For this review, take the finished solid that the model builds, in its own axes (mm). Face numbers are marked on the shaded views. A direction names the side the tool comes from. Give positions to 0.01 mm unless a question says otherwise; leave off trailing zeros. Loops run counter-clockwise (first coordinate to the right, second up) from the corner with the lowest first, then second, coordinate; pieces in that order, holes last. Notation, with made-up numbers: (-19, 74.5) - (30, 74.5) arc R31 cw to (30, 107.5) - close; hole circle Ø8 at (-10.75, -33.75). An arc over 180 degrees is marked (long way). Use CSV: the item, a comma, the result in double quotes. Start each with the question number.
1. For the marked faces 1, 2 and 3, list the 3-axis set-ups (+Z, -Z, +X, -X, +Y, -Y) from which the entire face can be reached by the end or side of a thin tool; tool diameter is ignored.
2. Take a section at B-B on x = -6.5. Give the boundary of the cut face in (y, z).
3. Take a section at A-A on z = 1.5. Give the boundary of the cut face in (x, y), plus the area to 3 significant figures.
4. Take a section at D-D on z = -1.5. Give the boundary of the cut face in (x, y), plus the area to 3 significant figures.
5. Wall thickness on line 1 (X direction, y = -4, z = -1.9); line 2 (Y direction, x = 7, z = 2.05); line 3 (X direction, y = -3.75, z = 0.25): over which ranges is each line inside the solid? List them lowest first.
6. Take a section at C-C on y = -3.5. Give the boundary of the cut face in (x, z).
7. For pin 1 (2.5 mm diameter, centred on x = -7, y = -4, fed in from -Z); pin 2 (3 mm diameter, centred on x = 9, y = -2.5, fed in from +Z); pin 3 (3 mm diameter, centred on x = 6, y = -4, fed in from +Z); pin 4 (2.5 mm diameter, centred on x = -7, y = -4, fed in from +Z), all flat-tipped, find the tip position at first contact; note any pin that passes through.
```python
from build123d import *

# Parameters (mm, degrees)
F1_DEPTH = 8
F3_D     = 2
F3_DEPTH = 0.6618861731
F4_D     = 2
F5_DEPTH = 1.5


with BuildPart() as f1:
    # F0 (on Front) → F1 (new body)
    with BuildSketch(Plane.XZ):
        with BuildLine():
            ThreePointArc((0.1467019637, 3.2967375591), (2.6022180015, 2.0293992886), (3.2331454446, -0.6608861731))
            Line((3.2331454446, -0.6608861731), (10.2443375631, -0.6608861731))
            Line((10.2443375631, -0.6608861731), (10.2443375631, 3.2967375591))
            Line((10.2443375631, 3.2967375591), (7.589418496, 3.2967375591))
            ThreePointArc((7.589418496, 3.2967375591), (5.7792360743, 3.6359179316), (4.2146449918, 4.6074417191))
            ThreePointArc((4.2146449918, 4.6074417191), (0, 6.2443375631), (-4.2146449918, 4.6074417191))
            ThreePointArc((-4.2146449918, 4.6074417191), (-5.7792360743, 3.6359179316), (-7.589418496, 3.2967375591))
            Line((-7.589418496, 3.2967375591), (-10.2443375631, 3.2967375591))
            Line((-10.2443375631, 3.2967375591), (-10.2443375631, -0.6608861731))
            Line((-10.2443375631, -0.6608861731), (-3.2331454446, -0.6608861731))
            ThreePointArc((-3.2331454446, -0.6608861731), (-2.6022180015, 2.0293992886), (-0.1467019637, 3.2967375591))
            ThreePointArc((-0.1467019637, 3.2967375591), (0, 3.3), (0.1467019637, 3.2967375591))
        make_face()
    extrude(amount=F1_DEPTH)

    # F3 (through all, one way)
    with BuildSketch(Plane.XY):
        with Locations((-7, -4), (7, -4)):
            Circle(F3_D / 2)
    extrude(amount=-F3_DEPTH, mode=Mode.SUBTRACT)

    # F4 (through all)
    with Locations(Plane(origin=(0, 0, 0), x_dir=(1, 0, 0), z_dir=(0, 0, -1))):
        with Locations((-7, 4), (7, 4)):
            Hole(F4_D / 2)

    # F5 (add): faces of the model
    f5_faces = [f1.faces().sort_by_distance(p)[0] for p in [
        (3.3395206367, -4, -0.6608861731),
        (-10.137962371, -4, -0.6608861731),
    ]]
    extrude(f5_faces, amount=F5_DEPTH)


solid = f1.part
```
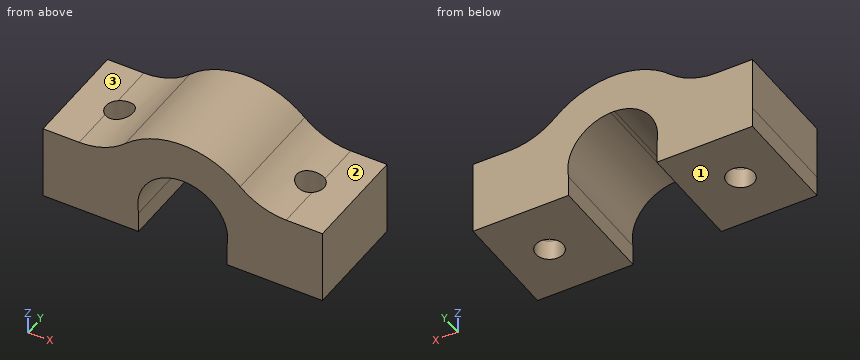
Check result:
1,face 1,"-Z, +X, -X, +Y, -Y"
1,face 2,"+Z, +X, +Y, -Y"
1,face 3,"+Z, -X, +Y, -Y"
2,outline,"(-8, -2.16) - (-4.87, -2.16) - (-4.87, 3.42) - (-8, 3.42) - close; (-3.13, -2.16) - (0, -2.16) - (0, 3.42) - (-3.13, 3.42) - close"
3,outline,"(-10.24, -8) - (-2.94, -8) - (-2.94, 0) - (-10.24, 0) - close; (2.94, -8) - (10.24, -8) - (10.24, 0) - (2.94, 0) - close; hole circle Ø2 at (-7, -4); hole circle Ø2 at (7, -4)"
3,area,"111 mm²"
4,outline,"(-10.24, -8) - (-3.23, -8) - (-3.23, 0) - (-10.24, 0) - close; (3.23, -8) - (10.24, -8) - (10.24, 0) - (3.23, 0) - close; hole circle Ø2 at (-7, -4); hole circle Ø2 at (7, -4)"
4,area,"106 mm²"
5,line 1,"x = -10.24 to -8, -6 to -3.23, 3.23 to 6, 8 to 10.24"
5,line 2,"y = -8 to -5, -3 to 0"
5,line 3,"x = -10.24 to -7.97, -6.03 to -3.29, 3.29 to 6.03, 7.97 to 10.24"
6,outline,"(-10.24, -2.16) - (-7.87, -2.16) - (-7.87, 3.3) - (-10.24, 3.3) - close; (-6.13, -2.16) - (-3.23, -2.16) - (-3.23, -0.66) arc R3.3 cw (long way) to (3.23, -0.66) - (3.23, -2.16) - (6.13, -2.16) - (6.13, 3.51) arc R5 cw to (4.21, 4.61) arc R6.24 ccw to (-4.21, 4.61) arc R5 cw to (-6.13, 3.51) - close; (7.87, -2.16) - (10.24, -2.16) - (10.24, 3.3) - (7.87, 3.3) - close"
7,pin 1,"stops at z = -2.16"
7,pin 2,"stops at z = 3.3"
7,pin 3,"stops at z = 4.37"
7,pin 4,"stops at z = 3.65"
